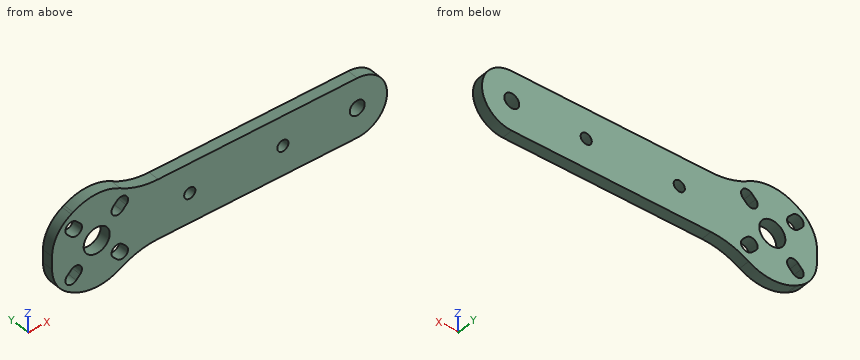
```python
from build123d import *

# Parameters (mm, degrees)
EXTRUDE_1_DEPTH     = 3
SKETCH_8_R          = 12.5
EXTRUDE_2_DEPTH     = 3
SKETCH_2_R          = 3.5
CUT_EXTRUDE_1_DEPTH = 159.522080481
SKETCH_5_R          = 1.5
CUT_EXTRUDE_2_DEPTH = 159.522080481
FILLET_3_R          = 20
SKETCH_9_R          = 2
CUT_EXTRUDE_3_DEPTH = 159.522080481
SKETCH_12_W         = 86.588173056
SKETCH_12_H         = 26.208680734
CUT_EXTRUDE_4_DEPTH = 159.522080481
FILLET_4_R          = 10
SKETCH_13_R         = 1.5
CUT_EXTRUDE_5_DEPTH = 159.522080481


with BuildPart() as part:
    # 草图1 → 凸台-拉伸1 (new body)
    with BuildSketch(Plane(origin=(0, 0, 0), x_dir=(1, 0, 0), z_dir=(0, 1, 0))):
        with BuildLine():
            Line((0, 8), (150, 8))
            ThreePointArc((150, 8), (158, 0), (150, -8))
            Line((150, -8), (0, -8))
            ThreePointArc((0, -8), (-8, 0), (0, 8))
        make_face()
    extrude(amount=EXTRUDE_1_DEPTH)

    # 草图8 → 凸台-拉伸2 (add)
    with BuildSketch(Plane(origin=(0, 3, 0), x_dir=(1, 0, 0), z_dir=(0, 1, 0))):
        with Locations((80, 0)):
            Circle(SKETCH_8_R)
    extrude(amount=-EXTRUDE_2_DEPTH)

    # 草图2 → 切除-拉伸1 (cut, through all)
    with BuildSketch(Plane(origin=(0, 3, 0), x_dir=(1, 0, 0), z_dir=(0, 1, 0))):
        with Locations(Location((80, 0, 0), (0, 0, 270))):
            Circle(SKETCH_2_R)
        with BuildLine():
            Line((84.456249475, 6.857459024), (85.516909647, 7.918119195))
            ThreePointArc((85.516909647, 7.918119195), (87.918119195, 7.918119195), (87.918119195, 5.516909647))
            Line((87.918119195, 5.516909647), (86.857459024, 4.456249475))
            ThreePointArc((86.857459024, 4.456249475), (84.456249475, 4.456249475), (84.456249475, 6.857459024))
        make_face()
        with BuildLine():
            Line((84.456249475, -6.857459024), (85.516909647, -7.918119195))
            ThreePointArc((85.516909647, -7.918119195), (87.918119195, -7.918119195), (87.918119195, -5.516909647))
            Line((87.918119195, -5.516909647), (86.857459024, -4.456249475))
            ThreePointArc((86.857459024, -4.456249475), (84.456249475, -4.456249475), (84.456249475, -6.857459024))
        make_face()
        with BuildLine():
            Line((73.142540976, -4.456249475), (72.081880805, -5.516909647))
            ThreePointArc((72.081880805, -5.516909647), (72.081880805, -7.918119195), (74.483090353, -7.918119195))
            Line((74.483090353, -7.918119195), (75.543750525, -6.857459024))
            ThreePointArc((75.543750525, -6.857459024), (75.543750525, -4.456249475), (73.142540976, -4.456249475))
        make_face()
        with BuildLine():
            Line((75.543750525, 6.857459024), (74.483090353, 7.918119195))
            ThreePointArc((74.483090353, 7.918119195), (72.081880805, 7.918119195), (72.081880805, 5.516909647))
            Line((72.081880805, 5.516909647), (73.142540976, 4.456249475))
            ThreePointArc((73.142540976, 4.456249475), (75.543750525, 4.456249475), (75.543750525, 6.857459024))
        make_face()
    extrude(amount=-CUT_EXTRUDE_1_DEPTH, mode=Mode.SUBTRACT)

    # 草图5 → 切除-拉伸2 (cut, through all)
    with BuildSketch(Plane(origin=(0, 3, 0), x_dir=(1, 0, 0), z_dir=(0, 1, 0))):
        with Locations(Location((10, 0, 0), (0, 0, 270))):
            Circle(SKETCH_5_R)
        with Locations(Location((0, 5, 0), (0, 0, 270))):
            Circle(SKETCH_5_R)
        with Locations(Location((0, -5, 0), (0, 0, 270))):
            Circle(SKETCH_5_R)
    extrude(amount=-CUT_EXTRUDE_2_DEPTH, mode=Mode.SUBTRACT)

    # 圆角3
    fillet_3_edges = [part.edges().sort_by_distance(p)[0] for p in [
        (70.395313644, 1.5, 8),
        (70.395313644, 1.5, -8),
        (89.604686356, 1.5, 8),
        (89.604686356, 1.5, -8),
    ]]
    fillet(fillet_3_edges, radius=FILLET_3_R)

    # 草图9 → 切除-拉伸3 (cut, through all)
    with BuildSketch(Plane(origin=(0, 3, 0), x_dir=(1, 0, 0), z_dir=(0, 1, 0))):
        with Locations(Location((150, 0, 0), (0, 0, 270))):
            Circle(SKETCH_9_R)
    extrude(amount=-CUT_EXTRUDE_3_DEPTH, mode=Mode.SUBTRACT)

    # 草图12 → 切除-拉伸4 (cut, through all)
    with BuildSketch(Plane(origin=(0, 3, 0), x_dir=(1, 0, 0), z_dir=(0, 1, 0))):
        with Locations((24.705913472, 0)):
            Rectangle(SKETCH_12_W, SKETCH_12_H)
    extrude(amount=-CUT_EXTRUDE_4_DEPTH, mode=Mode.SUBTRACT)

    # 圆角4
    fillet_4_edges = [part.edges().sort_by_distance(p)[0] for p in [
        (68, 1.5, -8.51282473),
        (68, 1.5, 8.51282473),
    ]]
    fillet(fillet_4_edges, radius=FILLET_4_R)

    # 草图13 → 切除-拉伸5 (cut, through all)
    with BuildSketch(Plane(origin=(0, 3, 0), x_dir=(1, 0, 0), z_dir=(0, 1, 0))):
        with Locations(Location((105, 0, 0), (0, 0, 270))):
            Circle(SKETCH_13_R)
        with Locations(Location((130, 0, 0), (0, 0, 270))):
            Circle(SKETCH_13_R)
    extrude(amount=-CUT_EXTRUDE_5_DEPTH, mode=Mode.SUBTRACT)


solid = part.part
```
Input: part model. Units: mm. Frame: model coordinates. Coordinates: 2 decimals unless noted, no trailing zeros. Write each loop counter-clockwise with the first axis right and the second up, starting at its lowest first coordinate (ties: lowest second). Pieces come first, ordered by that corner, then holes.
1) Material intervals for line 1 along X through (y, z) = (1.35, 0); line 2 along Z through (x, y) = (105, 0.75); line 3 along Z through (x, y) = (150, 1.9), sorted ascending.
2) Pin query (flat end, axial travel): pin 1 Ø1.5 at (x, y) = (129, 1.5) entering from +Z; pin 2 Ø1.5 at (y, z) = (0.5, 2.5) entering from +X; pin 3 Ø1 at (x, y) = (109.5, 2.5) entering from -Z. Return the tip coordinate at first contact, or that it passes through.
3) Section A-A on x = 80. Output: boundary loops of the cut face in (y, z).
4) Section C-C on y = 1.9. State how many separate pieces and enclosed holes the cut face has, and give its area (3 significant figures).
5) Section D-D on x = 105. Output: boundary loops of the cut face in (y, z).
6) Section B-B on z = 0. Output: boundary loops of the cut face in (x, y), and give its area (3 significant figures).
Check result:
1. line 1: x = 68 to 76.5, 83.5 to 103.5, 106.5 to 128.5, 131.5 to 148, 152 to 158
1. line 2: z = -8 to -1.5, 1.5 to 8
1. line 3: z = -8 to -2, 2 to 8
2. pin 1: stops at z = 8
2. pin 2: stops at x = 157.81
2. pin 3: stops at z = -8
3. outline: (0, -12.5) - (3, -12.5) - (3, -3.5) - (0, -3.5) - close; (0, 3.5) - (3, 3.5) - (3, 12.5) - (0, 12.5) - close
4. separate pieces: 1
4. enclosed holes: 8
4. area: 1,410 mm2
5. outline: (0, -8) - (3, -8) - (3, -1.5) - (0, -1.5) - close; (0, 1.5) - (3, 1.5) - (3, 8) - (0, 8) - close
6. outline: (68, 0) - (76.5, 0) - (76.5, 3) - (68, 3) - close; (83.5, 0) - (103.5, 0) - (103.5, 3) - (83.5, 3) - close; (106.5, 0) - (128.5, 0) - (128.5, 3) - (106.5, 3) - close; (131.5, 0) - (148, 0) - (148, 3) - (131.5, 3) - close; (152, 0) - (158, 0) - (158, 3) - (152, 3) - close
6. area: 219 mm2
